For this review, take the finished solid that the model builds, in its own axes (mm). A direction names the side the tool comes from. Give positions to 0.01 mm unless a question says otherwise; leave off trailing zeros. Order: outer loops, then holes, each group sorted by start corner. A loop starts at its lowest first (then second) coordinate and runs counter-clockwise, first axis right, second up. Notation, with made-up numbers: M 73.5,-36.5 L 128.5,-36.5 A26 cw 128.5,-7.5 Z; hole C -4.5,38 d8. An arc over 180 degrees is marked long. Answer as CSV lines item,"result". Start each with the question number.
1. We need section C-C, the plane z = -1. Give the boundary of the cut face in (x, y).
2. For line 1 along Z through (x, y) = (2.5, 1.75); line 2 along Y through (x, z) = (-0.75, 0.75); line 3 along Y through (x, z) = (-0.25, -1.5), list the stretches that pass through material, from the lowest coordinate up.
3. Machinability: for faces 1 (the conical face through (-0.007, 3.644, 2.672)), 2 (the flat face through (-2, -2, 0)), which of the approach directions +Z, -Z, +X, -X, +Y, -Y give a long, thin tool a straight path to every point of the face, cutting with its end or side? Answer none if there is none.
4. We need section B-B, the plane y = 0. Give the boundary of the cut face in (x, z).
5. Clearance check with flat-ended pins moving along their axes: P1, Ø1, axis at x = 1, z = 1, coming from the +Y side; P2, Ø1, axis at x = -2, z = -6, coming from the +Y side; P3, Ø3, axis at y = 2, z = -2.5, coming from the +X side. State where each tip first meets the part, or that it passes through.
6. We need section A-A, the plane z = 1.75. Give the boundary of the cut face in (x, y), and give its area (3 significant figures).
from build123d import *

# Parameters (mm, degrees)
EXTRUDE_1_DEPTH = 2.8
SKETCH_2_R      = 2
EXTRUDE_2_DEPTH = 7.2
CHAMFER_1_SIZE  = 0.75


with BuildPart() as part:
    # Эскиз1 → Вытянуть1 (new body)
    with BuildSketch(Plane.XY):
        Polygon((0, 4.041451884), (-3.5, 2.020725942), (-3.5, -2.020725942), (0, -4.041451884), (3.5, -2.020725942), (3.5, 2.020725942), align=None)
    extrude(amount=EXTRUDE_1_DEPTH)

    # Эскиз2 → Вытянуть2 (add)
    with BuildSketch(Plane(origin=(0, 0, 0), x_dir=(-1, 0, 0), z_dir=(0, 0, -1))):
        Circle(SKETCH_2_R)
    extrude(amount=EXTRUDE_2_DEPTH)

    # Эскиз15 → Вырез-Повернуть1 (revolve, cut)
    with BuildSketch(Plane(origin=(0, 0, 0), x_dir=(0, 0, -1), z_dir=(1, 0, 0))):
        Polygon((-2.8, 4.041451884), (-2.8, 3.516451884), (-2.275, 4.041451884), align=None)
    revolve(axis=Axis((0, 0, 5.265296569), (0, 0, -1)), mode=Mode.SUBTRACT)

    # Фаска1
    chamfer_1_edges = [part.edges().sort_by_distance(p)[0] for p in [
        (2, 0, -7.2),
    ]]
    chamfer(chamfer_1_edges, length=CHAMFER_1_SIZE)


solid = part.part
Result set:
1,outline,"C 0,0 d4"
2,line 1,"0 to 2.8"
2,line 2,"-3.61 to 3.61"
2,line 3,"-1.98 to 1.98"
3,face 1,"+Z, +Y"
3,face 2,"-Z"
4,outline,"M -3.5,0 L -2,0 L -2,-6.45 L -1.25,-7.2 L 1.25,-7.2 L 2,-6.45 L 2,0 L 3.5,0 L 3.5,2.8 L -3.5,2.8 Z"
5,P1,"y = 3.75"
5,P2,"y = 1.32"
5,P3,"x = 1.94"
6,outline,"M -3.5,-2.02 L 0,-4.04 L 3.5,-2.02 L 3.5,2.02 L 0,4.04 L -3.5,2.02 Z"
6,area,"42.4 mm2"
